from build123d import *

# Parameters (mm, degrees)
SKETCH1_R           = 2
BOSS_EXTRUDE1_DEPTH = 3
SKETCH2_R           = 2
CUT_EXTRUDE1_DEPTH  = 110.604839186
FILLET1_R           = 2


with BuildPart() as part:
    # Sketch1 → Boss-Extrude1 (new body)
    with BuildSketch(Plane.XY):
        Polygon((78.713203436, 49.493203436), (57.5, 28.28), (57.5, -28.28), (78.713203436, -49.493203436), (51.993203436, -76.213203436), (30.78, -55), (-30.78, -55), (-51.993203436, -76.213203436), (-78.713203436, -49.493203436), (-57.5, -28.28), (-57.5, 28.28), (-78.713203436, 49.493203436), (-51.993203436, 76.213203436), (-30.78, 55), (30.78, 55), (51.993203436, 76.213203436), align=None)
        with Locations((29, -24.5)):
            Circle(SKETCH1_R, mode=Mode.SUBTRACT)
        with Locations((29, 24.5)):
            Circle(SKETCH1_R, mode=Mode.SUBTRACT)
        with Locations((-29, -24.5)):
            Circle(SKETCH1_R, mode=Mode.SUBTRACT)
        with Locations((-29, 24.5)):
            Circle(SKETCH1_R, mode=Mode.SUBTRACT)
    extrude(amount=BOSS_EXTRUDE1_DEPTH)

    # Sketch2 → Cut-Extrude1 (cut, through all)
    with BuildSketch(Plane.XY.offset(3)):
        with Locations((43.079339828, 53.30726189)):
            Circle(SKETCH2_R)
        with Locations((53.685941546, 63.913863607)):
            Circle(SKETCH2_R)
        with Locations((55.80726189, 40.579339828)):
            Circle(SKETCH2_R)
        with Locations((66.413863607, 51.185941546)):
            Circle(SKETCH2_R)
        with Locations((-66.413863607, -51.185941546)):
            Circle(SKETCH2_R)
        with Locations((-55.80726189, -40.579339828)):
            Circle(SKETCH2_R)
        with Locations((-43.079339828, -53.30726189)):
            Circle(SKETCH2_R)
        with Locations((-53.685941546, -63.913863607)):
            Circle(SKETCH2_R)
        with Locations((-55.948736265, 64.468991324)):
            Circle(SKETCH2_R)
        with Locations((-42.524212111, 51.044467171)):
            Circle(SKETCH2_R)
        with Locations((-53.130813829, 40.437865453)):
            Circle(SKETCH2_R)
        with Locations((-66.555337983, 53.862389606)):
            Circle(SKETCH2_R)
        with Locations((55.600435219, -40.786166499)):
            Circle(SKETCH2_R)
        with Locations((42.872513157, -53.51408856)):
            Circle(SKETCH2_R)
        with Locations((66.207036937, -51.392768217)):
            Circle(SKETCH2_R)
        with Locations((53.479114875, -64.120690278)):
            Circle(SKETCH2_R)
    extrude(amount=-CUT_EXTRUDE1_DEPTH, mode=Mode.SUBTRACT)

    # Fillet1
    fillet1_edges = [part.edges().sort_by_distance(p)[0] for p in [
        (78.713203436, -49.493203436, 1.5),
        (51.993203436, -76.213203436, 1.5),
        (-51.993203436, -76.213203436, 1.5),
        (-78.713203436, -49.493203436, 1.5),
        (-78.713203436, 49.493203436, 1.5),
        (-51.993203436, 76.213203436, 1.5),
        (51.993203436, 76.213203436, 1.5),
        (78.713203436, 49.493203436, 1.5),
    ]]
    fillet(fillet1_edges, radius=FILLET1_R)


solid = part.part
The model under review builds one solid part; all positions refer to its coordinate system, in mm. A direction names the side the tool comes from. Coordinates: 2 decimals unless noted, no trailing zeros. Loops run counter-clockwise (first coordinate to the right, second up) from the corner with the lowest first, then second, coordinate; pieces in that order, holes last.
(1) Wall thickness on L1, parallel to Y at x = -29, z = 2; L2, parallel to X at y = 18.5, z = 2.25; L3, parallel to X at y = 23.5, z = 1: over which ranges is each line inside the solid? List them lowest first.
Determined:
L1: y = -55 to -26.5, -22.5 to 22.5, 26.5 to 55
L2: x = -57.5 to 57.5
L3: x = -57.5 to -30.73, -27.27 to 27.27, 30.73 to 57.5
(2) Consider section A-A, the plane x = 29. Give the boundary of the cut face in (y, z).
Determined:
outline: (-55, 0) - (-26.5, 0) - (-26.5, 3) - (-55, 3) - close; (-22.5, 0) - (22.5, 0) - (22.5, 3) - (-22.5, 3) - close; (26.5, 0) - (55, 0) - (55, 3) - (26.5, 3) - close
(3) Consider section D-D, the plane z = 0.45. Give the number of separate pieces and of enclosed holes in the cut face, plus the area to 3 significant figures.
Determined:
separate pieces: 1
enclosed holes: 20
area: 15,500 mm2
(4) Tool access review of faces 1 (the cylindrical face through (-27.092, -23.899, 1.479)), 2 (the flat face through (-67.26, 38.04, 1.48)), 3 (the flat face through (-40.82, 65.04, 1.48)): name each direction out of +Z, -Z, +X, -X, +Y, -Y from which nothing blocks a thin tool from reaching the whole face with its end or side.
Determined:
face 1: +Z, -Z
face 2: +Z, -Z, -X
face 3: +Z, -Z, +Y
(5) Draft analysis for pull direction X (two halves, no side actions). For faces 4 (the flat face through (1, 1, 0)), 5 (the cylindrical face through (57.51, -40.19, 1.52)), 6 (the flat face through (-65.52, 62.686, 1.479)), state which applies: +X half, -X half, draft (parallel to the pull), parting line (faces both ways), or undercut.
Determined:
face 4: draft
face 5: undercut
face 6: -X half
(6) Insertion check: P1, Ø2.5, axis at x = -55.81, y = -40.58, coming from the +Z side; P2, Ø0.9, axis at y = 3, z = 2, coming from the -X side; P3, Ø1.5, axis at y = 47.5, z = 1, coming from the -X side. Each pin has a flat end and moves straight along its axis. Give the tip position at first contact, or say it passes through.
Determined:
P1: passes through
P2: stops at x = -57.5
P3: stops at x = -77.45
(7) Consider section C-C, the plane x = -21. Give the boundary of the cut face in (y, z), plus the area to 3 significant figures.
Determined:
outline: (-55, 0) - (55, 0) - (55, 3) - (-55, 3) - close
area: 330 mm2
(8) Consider section B-B, the plane y = -24.5. Give the boundary of the cut face in (x, z), plus the area to 3 significant figures.
Determined:
outline: (-57.5, 0) - (-31, 0) - (-31, 3) - (-57.5, 3) - close; (-27, 0) - (27, 0) - (27, 3) - (-27, 3) - close; (31, 0) - (57.5, 0) - (57.5, 3) - (31, 3) - close
area: 321 mm2
